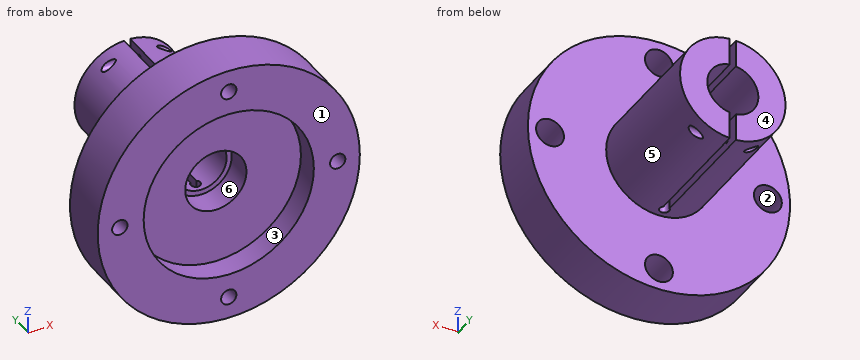
```python
from build123d import *

# Parameters (mm, degrees)
CUT_EXTRUDE1_DEPTH      = 39.5
CUT_EXTRUDE1_DEPTH_BACK = 39.5
CUT_EXTRUDE2_START      = -2.5
SKETCH3_R               = 1.25
CUT_EXTRUDE2_DEPTH      = 36.1
SKETCH4_R               = 0.5
CUT_EXTRUDE3_DEPTH      = 42.9
SKETCH5_R               = 2.25
CUT_EXTRUDE4_DEPTH      = 56.0000001
SKETCH6_R               = 4.1
CUT_EXTRUDE5_DEPTH      = 9
CIRPATTERN1_COUNT       = 4


with BuildPart() as part:
    # Sketch1 → Revolve1 (revolve)
    with BuildSketch(Plane.XY):
        Polygon((7.5, 55), (7.5, 15), (9, 15), (9, 7), (25, 7), (25, 0), (38.5, 0), (38.5, 15), (15.5, 15), (15.5, 55), align=None)
    revolve(axis=Axis((0, 0, 0), (0, 1, 0)))

    # Sketch2 → Cut-Extrude1 (cut, two sides)
    with BuildSketch(Plane.XY) as cut_extrude1_sk:
        with BuildLine():
            Line((-0.9, 55), (0.9, 55))
            Line((0.9, 55), (0.9, 19.072380529))
            ThreePointArc((0.9, 19.072380529), (0, 16.6), (-0.9, 19.072380529))
            Line((-0.9, 19.072380529), (-0.9, 55))
        make_face()
    extrude(amount=CUT_EXTRUDE1_DEPTH, mode=Mode.SUBTRACT)
    extrude(cut_extrude1_sk.sketch, amount=-CUT_EXTRUDE1_DEPTH_BACK, mode=Mode.SUBTRACT)

    # Sketch3 → Cut-Extrude2 (cut, through all)
    with BuildSketch(Plane(origin=(-0.9, 0, 0), x_dir=(0, 0, -1), z_dir=(1, 0, 0)).offset(CUT_EXTRUDE2_START)):
        with Locations((-13, 50)):
            Circle(SKETCH3_R)
        with Locations((13, 50)):
            Circle(SKETCH3_R)
    cut_extrude2 = extrude(amount=-CUT_EXTRUDE2_DEPTH, mode=Mode.SUBTRACT)

    # Sketch4 → Cut-Extrude3 (cut, through all)
    with BuildSketch(Plane.ZY.offset(3.4)):
        with Locations((13, 50)):
            Circle(SKETCH4_R)
        with Locations((-13, 50)):
            Circle(SKETCH4_R)
    extrude(amount=-CUT_EXTRUDE3_DEPTH, mode=Mode.SUBTRACT)

    # Mirror1: Cut-Extrude2 across plane
    add(cut_extrude2.mirror(Plane(origin=(0, 0, 0), x_dir=(0, 0, 1), z_dir=(1, 0, 0))), mode=Mode.SUBTRACT)

    # Sketch5 → Cut-Extrude4 (cut, through all)
    with BuildSketch(Plane.XZ):
        with Locations((32, 0)):
            Circle(SKETCH5_R)
    cut_extrude4 = extrude(amount=-CUT_EXTRUDE4_DEPTH, mode=Mode.SUBTRACT)

    # Sketch6 → Cut-Extrude5 (cut)
    with BuildSketch(Plane(origin=(0, 15, 0), x_dir=(1, 0, 0), z_dir=(0, 1, 0))):
        with Locations((32, 0)):
            Circle(SKETCH6_R)
    cut_extrude5 = extrude(amount=-CUT_EXTRUDE5_DEPTH, mode=Mode.SUBTRACT)

    # CirPattern1: Cut-Extrude4, Cut-Extrude5 ×4 about axis
    cirpattern1_axis = Axis((0, 0, 0), (0, 1, 0))
    for i in range(1, CIRPATTERN1_COUNT):
        add(cut_extrude4.rotate(cirpattern1_axis, i * 360 / CIRPATTERN1_COUNT), mode=Mode.SUBTRACT)
        add(cut_extrude5.rotate(cirpattern1_axis, i * 360 / CIRPATTERN1_COUNT), mode=Mode.SUBTRACT)


solid = part.part
```
CAD build for the part. Positions are in the model's coordinates, mm. Face numbers are marked on the shaded views. A direction names the side the tool comes from. Round coordinates to 2 decimals unless told otherwise and drop trailing zeros. Loops run counter-clockwise (first coordinate to the right, second up) from the corner with the lowest first, then second, coordinate; pieces in that order, holes last. Notation, with made-up numbers: M 7.5,76.5 L 62.5,76.5 A24 ccw 62.5,115.5 Z; hole C 20,63.25 d5. An arc over 180 degrees is marked long. Use a Markdown table: item, result. Add a question column.
(1) Cut at D-D (x = 20.5). Give the cut face in (y, z), and give its area (3 significant figures).
(2) Flat gauge pins, fed straight in: pin 1 (8 mm diameter, centred on x = -27, y = 10, fed in from -Z); pin 2 (6 mm diameter, centred on y = 8, z = 23, fed in from +X); pin 3 (6 mm diameter, centred on x = -9.5, z = -7, fed in from -Y); pin 4 (9 mm diameter, centred on x = 0, z = 0.5, fed in from -Y). Where does each tip first touch, or does it go through?
(3) Pull direction Z, two halves, no side cores. Call the marked faces 4, 5 and 6: +Z half, -Z half, draft (parallel to the pull), parting line (faces both ways), or undercut.
(4) Drill centre lines: line 1 (Y direction, x = 10, z = 1.5); line 2 (Y direction, x = -28.5, z = 9); line 3 (X direction, y = 18, z = -13). Where is each one in solid material? Low to high.
(5) Cut at C-C (z = 0). State how many separate pieces and enclosed holes the cut face has, and give its area (3 significant figures).
(6) Which spindle directions (+Z, -Z, +X, -X, +Y, -Y) get a long thin tool onto all of the face, cutting with end or side? Do the marked faces 1, 2 and 3. Say none if no direction does.
(7) Cut at B-B (x = 32). Give the cut face in (y, z).
Geometry says:
| question | item | result |
|---|---|---|
| 1 | outline | M 0,-32.59 L 15,-32.59 L 15,32.59 L 0,32.59 L 0,14.31 L 7,14.31 L 7,-14.31 L 0,-14.31 Z |
| 1 | area | 777 mm² |
| 2 | pin 1 | stops at z = -30.87 |
| 2 | pin 2 | stops at x = 32.9 |
| 2 | pin 3 | stops at y = 7 |
| 2 | pin 4 | passes through |
| 3 | face 4 | draft |
| 3 | face 5 | parting line |
| 3 | face 6 | undercut |
| 4 | line 1 | y = 7 to 55 |
| 4 | line 2 | y = 0 to 15 |
| 4 | line 3 | x = -8.44 to -1.4, 1.4 to 8.44 |
| 5 | separate pieces | 4 |
| 5 | enclosed holes | 0 |
| 5 | area | 1,100 mm² |
| 6 | face 1 | +Z, -Z, +X, -X, -Y |
| 6 | face 2 | +Y |
| 6 | face 3 | -Y |
| 7 | outline | M 0,-21.41 L 15,-21.41 L 15,-4.1 L 6,-4.1 L 6,-2.25 L 0,-2.25 Z; M 0,2.25 L 6,2.25 L 6,4.1 L 15,4.1 L 15,21.41 L 0,21.41 Z |
